```python
from build123d import *

# Parameters (mm, degrees)
SKETCH1_R           = 2.1
BOSS_EXTRUDE1_DEPTH = 100
SKETCH_1_R          = 2.75
CUT_EXTRUDE_1_DEPTH = 102.469207152
SKETCH_2_R          = 2.75
CUT_EXTRUDE_2_DEPTH = 102.46920725


with BuildPart() as part:
    # Sketch1 → Boss-Extrude1 (new body)
    with BuildSketch(Plane(origin=(0, 0, 0), x_dir=(0, 0, -1), z_dir=(1, 0, 0))):
        with BuildLine():
            Line((-10, 9), (-10, 3))
            Line((-10, 3), (-8, 3))
            Line((-8, 3), (-8, 6))
            Line((-8, 6), (-7.060660172, 6))
            Line((-7.060660172, 6), (-4, 2.939339828))
            Line((-4, 2.939339828), (-4, -2.939339828))
            Line((-4, -2.939339828), (-7.060660172, -6))
            Line((-7.060660172, -6), (-8, -6))
            Line((-8, -6), (-8, -3))
            Line((-8, -3), (-10, -3))
            Line((-10, -3), (-10, -9))
            ThreePointArc((-10, -9), (-9.707106781, -9.707106781), (-9, -10))
            Line((-9, -10), (-3, -10))
            Line((-3, -10), (-3, -8))
            Line((-3, -8), (-6, -8))
            Line((-6, -8), (-6, -7.060660172))
            Line((-6, -7.060660172), (-2.939339828, -4))
            Line((-2.939339828, -4), (2.939339828, -4))
            Line((2.939339828, -4), (6, -7.060660172))
            Line((6, -7.060660172), (6, -8))
            Line((6, -8), (3, -8))
            Line((3, -8), (3, -10))
            Line((3, -10), (9, -10))
            ThreePointArc((9, -10), (9.707106781, -9.707106781), (10, -9))
            Line((10, -9), (10, -3))
            Line((10, -3), (8, -3))
            Line((8, -3), (8, -6))
            Line((8, -6), (7.060660172, -6))
            Line((7.060660172, -6), (4, -2.939339828))
            Line((4, -2.939339828), (4, 2.939339828))
            Line((4, 2.939339828), (7.060660172, 6))
            Line((7.060660172, 6), (8, 6))
            Line((8, 6), (8, 3))
            Line((8, 3), (10, 3))
            Line((10, 3), (10, 9))
            ThreePointArc((10, 9), (9.707106781, 9.707106781), (9, 10))
            Line((9, 10), (3, 10))
            Line((3, 10), (3, 8))
            Line((3, 8), (6, 8))
            Line((6, 8), (6, 7.060660172))
            Line((6, 7.060660172), (2.939339828, 4))
            Line((2.939339828, 4), (-2.939339828, 4))
            Line((-2.939339828, 4), (-6, 7.060660172))
            Line((-6, 7.060660172), (-6, 8))
            Line((-6, 8), (-3, 8))
            Line((-3, 8), (-3, 10))
            Line((-3, 10), (-9, 10))
            ThreePointArc((-9, 10), (-9.707106781, 9.707106781), (-10, 9))
        make_face()
        Circle(SKETCH1_R, mode=Mode.SUBTRACT)
    extrude(amount=BOSS_EXTRUDE1_DEPTH)

    # Sketch 1 → Cut-Extrude 1 (cut, through all)
    with BuildSketch(Plane(origin=(0, 4, 0), x_dir=(1, 0, 0), z_dir=(0, 1, 0))):
        with Locations(Location((41, -0.010660172, 0), (0, 0, 270))):
            Circle(SKETCH_1_R)
    extrude(amount=-CUT_EXTRUDE_1_DEPTH, mode=Mode.SUBTRACT)

    # Sketch 2 → Cut-Extrude 2 (cut, through all)
    with BuildSketch(Plane.XY.offset(4)):
        with Locations((59, -0.05)):
            Circle(SKETCH_2_R)
    extrude(amount=-CUT_EXTRUDE_2_DEPTH, mode=Mode.SUBTRACT)


solid = part.part
```
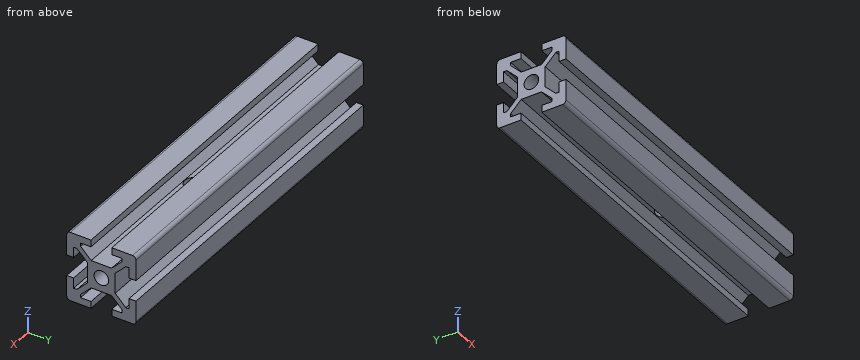
Geometry check sheet. Reference: the model listing, model coordinates, mm. Coordinates: 2 decimals unless noted, no trailing zeros. Write each loop counter-clockwise with the first axis right and the second up, starting at its lowest first coordinate (ties: lowest second). Pieces come first, ordered by that corner, then holes. Notation, with made-up numbers: (60, 30) -> (103, 30) arc R24 ccw to (103, 68) -> close; hole circle Ø3 at (48.25, -9.75). An arc over 180 degrees is marked (long way). Use CSV: the item, a comma, the result in double quotes. Start each with the question number.
Item 1: Thickness scan on line 1 (Y direction, x = 59, z = -0.5); line 2 (Y direction, x = 91, z = 8.75); line 3 (Z direction, x = 91, y = 4.5). Record the ranges inside material, lowest first.
Item 2: Depth check by flat-ended pin: pin 1 Ø1.5 at (x, z) = (86.5, -1.5) entering from +Y. Enter the tip coordinate at first touch or a pass-through.
Item 3: Cross-section at A-A, the plane z = 0. Record the cut outline in (x, y), plus the area to 3 significant figures.
Item 4: Cross-section at B-B, the plane y = -1. Record the cut outline in (x, z).
Answers:
1,line 1,"-4 to -2.8, 2.7 to 4"
1,line 2,"-10 to -3, 3 to 10"
1,line 3,"-10 to -8, -5.56 to -3.44, 3.44 to 5.56, 8 to 10"
2,pin 1,"y = 4"
3,outline,"(0, -4) -> (38.25, -4) -> (38.25, -2.1) -> (0, -2.1) -> close; (0, 2.1) -> (38.25, 2.1) -> (38.25, 4) -> (0, 4) -> close; (43.75, -4) -> (100, -4) -> (100, -2.1) -> (60.83, -2.1) arc R2.75 cw to (57.17, -2.1) -> (43.75, -2.1) -> close; (43.75, 2.1) -> (57.29, 2.1) arc R2.75 cw to (60.71, 2.1) -> (100, 2.1) -> (100, 4) -> (43.75, 4) -> close"
3,area,"356 mm^2"
4,outline,"(0, -4) -> (56.42, -4) -> (56.42, -1.85) -> (43.03, -1.85) arc R2.75 cw to (38.97, -1.85) -> (0, -1.85) -> close; (0, 1.85) -> (38.95, 1.85) arc R2.75 cw to (43.05, 1.85) -> (56.42, 1.85) -> (56.42, 4) -> (0, 4) -> close; (61.58, -4) -> (100, -4) -> (100, -1.85) -> (61.58, -1.85) -> close; (61.58, 1.85) -> (100, 1.85) -> (100, 4) -> (61.58, 4) -> close"
